CAD build for the part. Positions are in the model's coordinates, mm. Face numbers are marked on the shaded views. Coordinates: 2 decimals unless noted, no trailing zeros. Write each loop counter-clockwise with the first axis right and the second up, starting at its lowest first coordinate (ties: lowest second). Pieces come first, ordered by that corner, then holes. Notation, with made-up numbers: (44, -37) - (85, -37) arc R12 cw to (85, -23) - close; hole circle Ø6 at (-38.75, -11.75). An arc over 180 degrees is marked (long way). One line per question, with ' | ' between items. Start each with the question number.
1. Band-saw the part on C-C, the plane z = 4.5. Write the cut outline in (x, y).
2. Band-saw the part on A-A, the plane z = 58.5. Write the cut outline in (x, y), then the cut area to 4 significant figures.
3. Band-saw the part on B-B, the plane x = -93. Write the cut outline in (y, z).
4. Flat gauge pins, fed straight in: P1, Ø7.5, axis at x = -65.5, y = -148, coming from the +Z side; P2, Ø4.5, axis at x = -10.39, z = 65.5, coming from the +Y side; P3, Ø3, axis at y = -133.5, z = 6, coming from the +X side. Where does each tip first touch, or does it go through?
5. Probe line 1 (X direction, y = -197.5, z = 65.5); line 2 (X direction, y = -95.75, z = 16); line 3 (Y direction, x = -100, z = 28). List the from-to ranges inside material, lowest first.
6. Two-plate mould, pull along Y, no slides. Class the marked faces 1, 2 and 3: +Y half, -Y half, draft (parallel to the pull), parting line (faces both ways), or undercut.
7. Band-saw the part on D-D, the plane y = -78.5. Write the cut outline in (x, z).
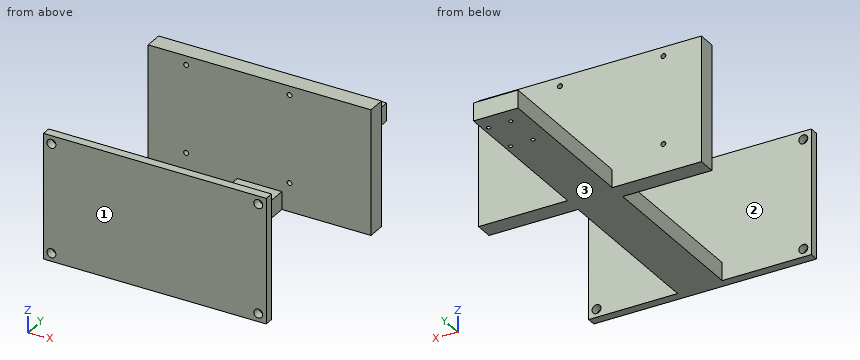
from build123d import *

# Parameters (mm, degrees)
SKETCH2_W           = 25
SKETCH2_H           = 90
SKETCH2_R           = 1.1
SKETCH2_H_2         = 10
SKETCH2_W_2         = 50
SKETCH2_H_3         = 100
BOSS_EXTRUDE3_DEPTH = 10
SKETCH5_W           = 125
SKETCH5_H           = 10
BOSS_EXTRUDE4_DEPTH = 60
SKETCH6_W           = 75
SKETCH6_H           = 5
BOSS_EXTRUDE5_DEPTH = 60
SKETCH8_W           = 10
SKETCH8_H           = 5
BOSS_EXTRUDE7_DEPTH = 50
SKETCH7_W           = 70
SKETCH7_H           = 5
BOSS_EXTRUDE8_DEPTH = 50
SKETCH12_R          = 2.5
CUT_EXTRUDE1_DEPTH  = 246.068129549
CUT_EXTRUDE2_REACH  = 186.752
SKETCH13_R          = 1.35


with BuildPart() as part:
    # Sketch2 → Boss-Extrude3 (new body)
    # profile 1 of 5: a face of its own
    with BuildSketch(Plane.XY):
        with Locations((-68.394568721, -43.658737525)):
            Rectangle(SKETCH2_W, SKETCH2_H)
        with Locations((-71.394568721, -29.020737525)):
            Circle(SKETCH2_R, mode=Mode.SUBTRACT)
        with Locations((-71.394568721, -8.020737525)):
            Circle(SKETCH2_R, mode=Mode.SUBTRACT)
        with Locations((-58.894568721, -29.020737525)):
            Circle(SKETCH2_R, mode=Mode.SUBTRACT)
        with Locations((-58.894568721, -8.020737525)):
            Circle(SKETCH2_R, mode=Mode.SUBTRACT)
    # profile 2 of 5: a face of its own
    with BuildSketch(Plane.XY):
        with Locations((-68.394568721, -93.658737525)):
            Rectangle(SKETCH2_W, SKETCH2_H_2)
    # profile 3 of 5: a face of its own
    with BuildSketch(Plane.XY):
        with Locations((-105.894568721, -93.658737525)):
            Rectangle(SKETCH2_W_2, SKETCH2_H_2)
    # profile 4 of 5: a face of its own
    with BuildSketch(Plane.XY):
        with Locations((-30.894568721, -93.658737525)):
            Rectangle(SKETCH2_W_2, SKETCH2_H_2)
    # profile 5 of 5: a face of its own
    with BuildSketch(Plane.XY):
        with Locations((-68.394568721, -148.658737525)):
            Rectangle(SKETCH2_W, SKETCH2_H_3)
    extrude(amount=BOSS_EXTRUDE3_DEPTH)

    # Sketch5 → Boss-Extrude4 (add)
    with BuildSketch(Plane.XY.offset(10)):
        with Locations((-68.394568721, -93.658737525)):
            Rectangle(SKETCH5_W, SKETCH5_H)
    extrude(amount=BOSS_EXTRUDE4_DEPTH)

    # Sketch6 → Boss-Extrude5 (add)
    with BuildSketch(Plane.XY.offset(10)):
        with Locations((-43.394568721, -196.158737525)):
            Rectangle(SKETCH6_W, SKETCH6_H)
    extrude(amount=BOSS_EXTRUDE5_DEPTH)

    # Sketch8 → Boss-Extrude7 (add)
    with BuildSketch(Plane(origin=(-55.894568721, 0, 0), x_dir=(0, 0, -1), z_dir=(1, 0, 0))):
        with Locations((-5, -196.158737525)):
            Rectangle(SKETCH8_W, SKETCH8_H)
    extrude(amount=BOSS_EXTRUDE7_DEPTH)

    # Sketch7 → Boss-Extrude8 (add)
    with BuildSketch(Plane.ZY.offset(80.894568721)):
        with Locations((35, -196.158737525)):
            Rectangle(SKETCH7_W, SKETCH7_H)
    extrude(amount=BOSS_EXTRUDE8_DEPTH)

    # Sketch12 → Cut-Extrude1 (cut, through all)
    with BuildSketch(Plane(origin=(0, -193.658737525, 0), x_dir=(1, 0, 0), z_dir=(0, 1, 0))):
        with Locations(Location((-126.394568721, -4.5, 0), (0, 0, 270))):
            Circle(SKETCH12_R)
        with Locations(Location((-126.394568721, -65.5, 0), (0, 0, 270))):
            Circle(SKETCH12_R)
        with Locations(Location((-10.394568721, -65.5, 0), (0, 0, 270))):
            Circle(SKETCH12_R)
        with Locations(Location((-10.394568721, -4.5, 0), (0, 0, 270))):
            Circle(SKETCH12_R)
    extrude(amount=-CUT_EXTRUDE1_DEPTH, mode=Mode.SUBTRACT)

    # Sketch13 → Cut-Extrude2 (cut, up to next)
    with BuildSketch(Plane(origin=(0, -88.658737525, 0), x_dir=(1, 0, 0), z_dir=(0, 1, 0)), mode=Mode.PRIVATE) as cut_extrude2_sk1:
        with Locations(Location((-109.594568721, -16, 0), (0, 0, 270))):
            Circle(SKETCH13_R)
    cut_extrude2_tool1 = extrude(cut_extrude2_sk1.sketch, amount=-CUT_EXTRUDE2_REACH, mode=Mode.PRIVATE) & part.part
    # Sketch13 → Cut-Extrude2 (cut, up to next)
    with BuildSketch(Plane(origin=(0, -88.658737525, 0), x_dir=(1, 0, 0), z_dir=(0, 1, 0)), mode=Mode.PRIVATE) as cut_extrude2_sk2:
        with Locations(Location((-109.594568721, -65, 0), (0, 0, 270))):
            Circle(SKETCH13_R)
    cut_extrude2_tool2 = extrude(cut_extrude2_sk2.sketch, amount=-CUT_EXTRUDE2_REACH, mode=Mode.PRIVATE) & part.part
    # Sketch13 → Cut-Extrude2 (cut, up to next)
    with BuildSketch(Plane(origin=(0, -88.658737525, 0), x_dir=(1, 0, 0), z_dir=(0, 1, 0)), mode=Mode.PRIVATE) as cut_extrude2_sk3:
        with Locations(Location((-51.594568721, -65, 0), (0, 0, 270))):
            Circle(SKETCH13_R)
    cut_extrude2_tool3 = extrude(cut_extrude2_sk3.sketch, amount=-CUT_EXTRUDE2_REACH, mode=Mode.PRIVATE) & part.part
    # Sketch13 → Cut-Extrude2 (cut, up to next)
    with BuildSketch(Plane(origin=(0, -88.658737525, 0), x_dir=(1, 0, 0), z_dir=(0, 1, 0)), mode=Mode.PRIVATE) as cut_extrude2_sk4:
        with Locations(Location((-51.594568721, -16, 0), (0, 0, 270))):
            Circle(SKETCH13_R)
    cut_extrude2_tool4 = extrude(cut_extrude2_sk4.sketch, amount=-CUT_EXTRUDE2_REACH, mode=Mode.PRIVATE) & part.part
    add(cut_extrude2_tool1.solids().sort_by_distance((-109.594569, -88.658738, 16))[0], mode=Mode.SUBTRACT)
    add(cut_extrude2_tool2.solids().sort_by_distance((-109.594569, -88.658738, 65))[0], mode=Mode.SUBTRACT)
    add(cut_extrude2_tool3.solids().sort_by_distance((-51.594569, -88.658738, 65))[0], mode=Mode.SUBTRACT)
    add(cut_extrude2_tool4.solids().sort_by_distance((-51.594569, -88.658738, 16))[0], mode=Mode.SUBTRACT)


solid = part.part
Filled in:
1) outline: (-130.89, -198.66) - (-128.89, -198.66) - (-128.89, -193.66) - (-130.89, -193.66) - close; (-130.89, -98.66) - (-80.89, -98.66) - (-80.89, -193.66) - (-123.89, -193.66) - (-123.89, -198.66) - (-12.89, -198.66) - (-12.89, -193.66) - (-55.89, -193.66) - (-55.89, -98.66) - (-5.89, -98.66) - (-5.89, -88.66) - (-55.89, -88.66) - (-55.89, 1.34) - (-80.89, 1.34) - (-80.89, -88.66) - (-130.89, -88.66) - close; (-7.89, -198.66) - (-5.89, -198.66) - (-5.89, -193.66) - (-7.89, -193.66) - close; hole circle Ø2.2 at (-71.39, -29.02); hole circle Ø2.2 at (-71.39, -8.02); hole circle Ø2.2 at (-58.89, -29.02); hole circle Ø2.2 at (-58.89, -8.02)
2) outline: (-130.89, -198.66) - (-5.89, -198.66) - (-5.89, -193.66) - (-130.89, -193.66) - close; (-130.89, -98.66) - (-5.89, -98.66) - (-5.89, -88.66) - (-130.89, -88.66) - close | area: 1,875 mm²
3) outline: (-198.66, 0) - (-193.66, 0) - (-193.66, 70) - (-198.66, 70) - close; (-98.66, 0) - (-88.66, 0) - (-88.66, 70) - (-98.66, 70) - close
4) P1: stops at z = 10 | P2: stops at y = -88.66 | P3: stops at x = -55.89
5) line 1: x = -130.89 to -128.89, -123.89 to -12.89, -7.89 to -5.89 | line 2: x = -130.89 to -110.94, -108.24 to -52.94, -50.24 to -5.89 | line 3: y = -198.66 to -193.66, -98.66 to -88.66
6) face 1: -Y half | face 2: undercut | face 3: draft
7) outline: (-80.89, 0) - (-55.89, 0) - (-55.89, 10) - (-80.89, 10) - close
